Answer from the drawing. Dimensions are ordinates in mm from the lowest x, y and z of the part. Give positions to 0.01 mm unless a question says otherwise; leave off trailing zeros. Loops run counter-clockwise (first coordinate to the right, second up) from the corner with the lowest first, then second, coordinate; pieces in that order, holes last. Notation, with made-up numbers: (26, 29.5) - (85, 29.5) arc R8 cw to (85, 43.5) - close; hole circle Ø3 at (-5, 23.25). An arc over 180 degrees is marked (long way). One line per question, with ' | ' between items. Start each with the question number.
1. Section D-D (z = 20) is taken. Determine the outline of the cut face in (x, y).
2. Section C-C (x = 53) is taken. Determine the outline of the cut face in (y, z).
3. Find the intervals of material crossed by line 1 (Z direction, x = 53, y = 1.6); line 2 (X direction, y = 3.9, z = 20); line 3 (Z direction, x = 151.5, y = 5.75), in increasing order.
4. Section B-B (z = 70.5) is taken. Determine the outline of the cut face in (x, y), plus the area to 3 significant figures.
5. This flat-tipped pin is pushed along its axis until it touches: pin 1 (6.5 mm diameter, centred on x = 153, z = 20, fed in from +Y). Where does it stop, or does it pass through?
6. Section A-A (y = 8) is taken. Determine the outline of the cut face in (x, z).
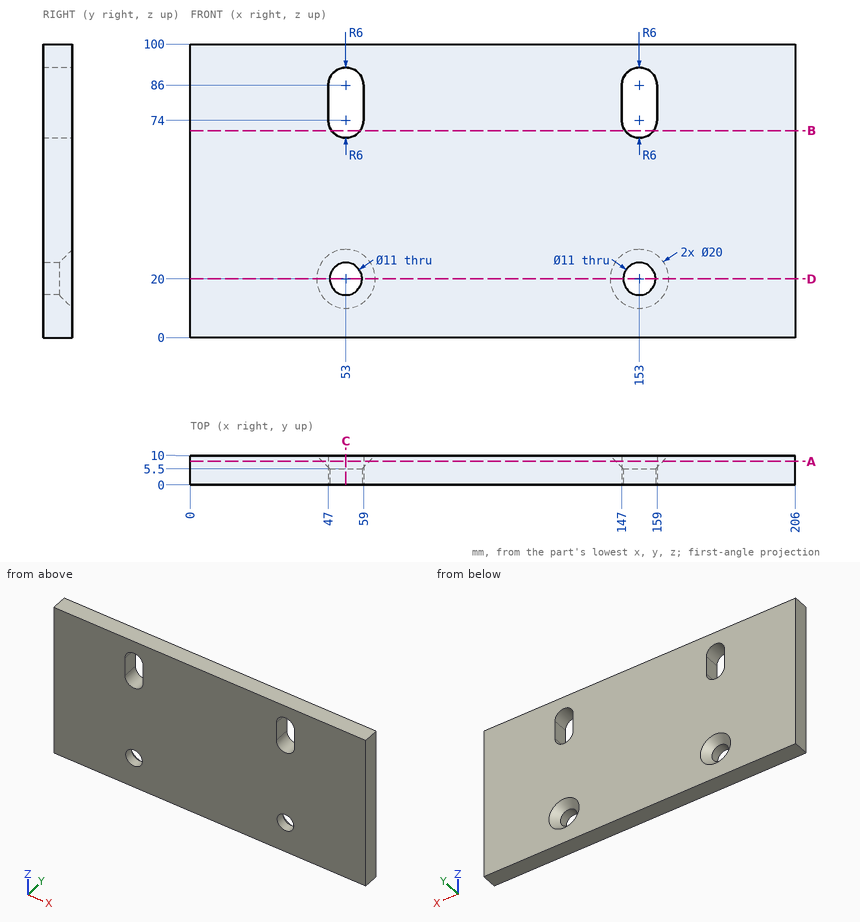
Conclusion:
1) outline: (0, 0) - (47.5, 0) - (47.5, 5.5) - (43, 10) - (0, 10) - close; (58.5, 0) - (147.5, 0) - (147.5, 5.5) - (143, 10) - (63, 10) - (58.5, 5.5) - close; (158.5, 0) - (206, 0) - (206, 10) - (163, 10) - (158.5, 5.5) - close
2) outline: (0, 0) - (10, 0) - (10, 10) - (5.5, 14.5) - (0, 14.5) - close; (0, 25.5) - (5.5, 25.5) - (10, 30) - (10, 68) - (0, 68) - close; (0, 92) - (10, 92) - (10, 100) - (0, 100) - close
3) line 1: 0 to 14.5, 25.5 to 68, 92 to 100 | line 2: 0 to 47.5, 58.5 to 147.5, 158.5 to 206 | line 3: 0 to 14.45, 25.55 to 68.19, 91.81 to 100
4) outline: (0, 0) - (48.13, 0) - (48.13, 10) - (0, 10) - close; (57.87, 0) - (148.13, 0) - (148.13, 10) - (57.87, 10) - close; (157.87, 0) - (206, 0) - (206, 10) - (157.87, 10) - close | area: 1,870 mm²
5) pin 1: through
6) outline: (0, 0) - (206, 0) - (206, 100) - (0, 100) - close; hole circle Ø16 at (53, 20); hole (47, 74) arc R6 ccw to (59, 74) - (59, 86) arc R6 ccw to (47, 86) - close; hole circle Ø16 at (153, 20); hole (147, 74) arc R6 ccw to (159, 74) - (159, 86) arc R6 ccw to (147, 86) - close
